from build123d import *

# Parameters (mm, degrees)
EXTRUDE_1_DEPTH     = 25
EXTRUDE_START       = -5
SKETCH_3_R          = 13.5
SKETCH_3_R_2        = 8
EXTRUDE_2_DEPTH     = 5
CUT_EXTRUDE_1_DEPTH = 58.063561053
SKETCH_5_W          = 10
SKETCH_5_H          = 14
EXTRUDE_3_DEPTH     = 11
SKETCH_6_W          = 15
SKETCH_6_H          = 13
EXTRUDE_4_DEPTH     = 10
SKETCH_7_W          = 10
SKETCH_7_H          = 14
CUT_EXTRUDE_2_DEPTH = 11
SKETCH_8_W          = 15
SKETCH_8_H          = 13
EXTRUDE_5_DEPTH     = 10
SKETCH_9_W          = 15
SKETCH_9_H          = 10
CUT_EXTRUDE_3_DEPTH = 3
EXTRUDE_6_DEPTH     = 25


with BuildPart() as part:
    # Эскиз1 → Бобышка-Вытянуть1 (new body)
    with BuildSketch(Plane.XY):
        with BuildLine():
            Line((-35, 25), (-35, -25))
            Line((-35, -25), (35, -25))
            Line((35, -25), (35, -12.5))
            Line((35, -12.5), (25, -12.5))
            Line((25, -12.5), (25, 12.5))
            Line((25, 12.5), (35, 12.5))
            Line((35, 12.5), (35, 25))
            Line((35, 25), (8, 25))
            ThreePointArc((8, 25), (0, 17), (-8, 25))
            Line((-8, 25), (-35, 25))
        make_face()
        Polygon((4, -19), (-4, -19), (-4, -4), (-4, 4), (0, 4), (0, -4), (4, -4), align=None, mode=Mode.SUBTRACT)
    extrude(amount=EXTRUDE_1_DEPTH)

    # Эскиз3 → Бобышка-Вытянуть2 (add)
    with BuildSketch(Plane.XY.offset(25).offset(EXTRUDE_START)):
        with Locations((0, 25)):
            Circle(SKETCH_3_R)
        with Locations((0, 25)):
            Circle(SKETCH_3_R_2, mode=Mode.SUBTRACT)
    extrude_2 = extrude(amount=EXTRUDE_2_DEPTH)

    # Эскиз4 → Вырез-Вытянуть1 (cut, through all)
    with BuildSketch(Plane.XZ.offset(-12.5)):
        Polygon((35, 25), (25, 0), (35, 0), align=None)
    extrude(amount=-CUT_EXTRUDE_1_DEPTH, mode=Mode.SUBTRACT)

    # Эскиз5 → Бобышка-Вытянуть3 (add)
    with BuildSketch(Plane.XY.offset(25)):
        with Locations((-30, 0)):
            Rectangle(SKETCH_5_W, SKETCH_5_H)
    extrude(amount=EXTRUDE_3_DEPTH)

    # Эскиз6 → Бобышка-Вытянуть4 (add)
    with BuildSketch(Plane(origin=(0, 0, 0), x_dir=(-1, 0, 0), z_dir=(0, 0, -1))):
        with Locations((42.5, 13.5)):
            Rectangle(SKETCH_6_W, SKETCH_6_H)
    extrude(amount=-EXTRUDE_4_DEPTH)

    # Эскиз7 → Вырез-Вытянуть2 (cut)
    with BuildSketch(Plane.XY.offset(36)):
        with Locations((-30, 0)):
            Rectangle(SKETCH_7_W, SKETCH_7_H)
    extrude(amount=-CUT_EXTRUDE_2_DEPTH, mode=Mode.SUBTRACT)

    # Эскиз8 → Бобышка-Вытянуть5 (add)
    with BuildSketch(Plane(origin=(0, 0, 0), x_dir=(-1, 0, 0), z_dir=(0, 0, -1))):
        with Locations((27.5, 0.5)):
            Rectangle(SKETCH_8_W, SKETCH_8_H)
    extrude(amount=EXTRUDE_5_DEPTH)

    # Эскиз9 → Вырез-Вытянуть3 (cut)
    with BuildSketch(Plane(origin=(0, 7, 0), x_dir=(1, 0, 0), z_dir=(0, 1, 0))):
        with Locations((-27.5, 5)):
            Rectangle(SKETCH_9_W, SKETCH_9_H)
    extrude(amount=-CUT_EXTRUDE_3_DEPTH, mode=Mode.SUBTRACT)

    # Эскиз10 → Бобышка-Вытянуть6 (add)
    with BuildSketch(Plane(origin=(0, 0, 0), x_dir=(-1, 0, 0), z_dir=(0, 0, -1))):
        Polygon((4, -19), (4, 4), (0, 4), (0, -4), (-4, -4), (-4, -19), align=None)
    extrude(amount=-EXTRUDE_6_DEPTH)

    # Зеркальное отражение1: Бобышка-Вытянуть2 across plane
    add(extrude_2.mirror(Plane(origin=(0, 0, 12.5), x_dir=(1, 0, 0), z_dir=(0, 0, -1))))


solid = part.part
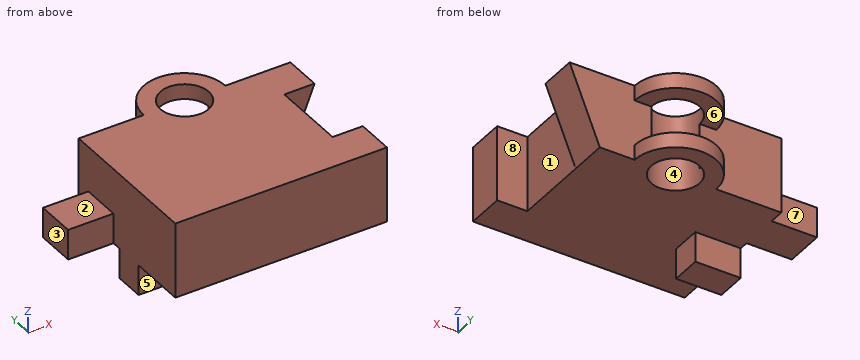
Geometry check sheet. Reference: the model listing, model coordinates, mm. Face numbers are marked on the shaded views. A direction names the side the tool comes from. Round coordinates to 2 decimals unless told otherwise and drop trailing zeros. Order: outer loops, then holes, each group sorted by start corner. A loop starts at its lowest first (then second) coordinate and runs counter-clockwise, first axis right, second up. Notation, with made-up numbers: M 47,-39.75 L 102,-39.75 A15 cw 102,-28.75 Z; hole C -3,23 d7. An arc over 180 degrees is marked long. Answer in a Markdown table with one row per item.
(1) Sectioned sample at B-B, the plane z = 3. Record the cut outline in (x, y), and give its area (3 significant figures).
Responses:
| item | result |
|---|---|
| outline | M -50,7 L -35,7 L -35,-25 L 35,-25 L 35,-12.5 L 25,-12.5 L 25,12.5 L 26.2,12.5 L 26.2,25 L 13.5,25 A13.5 ccw -13.5,25 L -35,25 L -35,20 L -50,20 Z; hole C 0,25 d16 |
| area | 3,420 mm² |
(2) Sectioned sample at A-A, the plane x = 0. Record the cut outline in (y, z).
Responses:
| item | result |
|---|---|
| outline | M -25,0 L 17,0 L 17,25 L -25,25 Z; M 33,0 L 38.5,0 L 38.5,5 L 33,5 Z; M 33,20 L 38.5,20 L 38.5,25 L 33,25 Z |
(3) Draft check along X on the marked faces 1, 2, 3 and 4. Enter one of: released by +X, released by -X, zero draft, split by the parting line, or undercut.
Responses:
| item | result |
|---|---|
| face 1 | released by +X |
| face 2 | zero draft |
| face 3 | released by -X |
| face 4 | undercut |
(4) Sectioned sample at D-D, the plane y = 31. Record the cut outline in (x, z), and give its area (3 significant figures).
Responses:
| item | result |
|---|---|
| outline | M -12.09,0 L -5.29,0 L -5.29,5 L -12.09,5 Z; M -12.09,20 L -5.29,20 L -5.29,25 L -12.09,25 Z; M 5.29,0 L 12.09,0 L 12.09,5 L 5.29,5 Z; M 5.29,20 L 12.09,20 L 12.09,25 L 5.29,25 Z |
| area | 136 mm² |
(5) Sectioned sample at C-C, the plane x = 30. Record the cut outline in (y, z).
Responses:
| item | result |
|---|---|
| outline | M -25,0 L -12.5,0 L -12.5,25 L -25,25 Z; M 12.5,12.5 L 25,12.5 L 25,25 L 12.5,25 Z |
(6) Go/stop test with flat-tipped pins: P1, Ø3, axis at x = -25, z = -6, coming from the -Y side; P2, Ø12, axis at x = -33.5, z = 8.5, coming from the +Y side; P3, Ø8, axis at y = 30.5, z = 8.5, coming from the -X side. Record where each tip stops, or that it passes through.
Responses:
| item | result |
|---|---|
| P1 | stops at y = -6 |
| P2 | stops at y = 25 |
| P3 | stops at x = -13.02 |
(7) Scan lines: probe 1 along Z at (x, y) = (-16.5, 3.5); probe 2 along Y at (x, z) = (-20.5, 7); probe 3 along Y at (x, z) = (0, 9.5). Record each from-to range of solid material in increasing order. Write a range as from..to.
Responses:
| item | result |
|---|---|
| probe 1 | z = 0..25 |
| probe 2 | y = -25..25 |
| probe 3 | y = -25..17 |
(8) Tool access check on the marked faces 5, 6, 7 and 8. Record the directions out of +Z, -Z, +X, -X, +Y, -Y that give a thin tool (end or side, any length) a straight path to the whole face; none if there is none.
Responses:
| item | result |
|---|---|
| face 5 | -Z, +X, -X, -Y |
| face 6 | +X, -X, +Y |
| face 7 | +Z, -Z, -X, +Y |
| face 8 | +Z, -Z, +X |
